Geometry check sheet. Reference: the model listing, model coordinates, mm. A direction names the side the tool comes from. Give positions to 0.01 mm unless a question says otherwise; leave off trailing zeros. Order: outer loops, then holes, each group sorted by start corner. A loop starts at its lowest first (then second) coordinate and runs counter-clockwise, first axis right, second up. Notation, with made-up numbers: M 59.25,4 L 89.25,4 A19 ccw 89.25,37 Z; hole C 2,-26.5 d9. An arc over 180 degrees is marked long. Put each result on its own line as item: value. Start each with the question number.
Q1. Section check C-C on y = -4.5. Record the cut outline in (x, z), then the cut area to 3 significant figures.
Q2. Access from +Z, -Z, +X, -X, +Y, -Y to the whole of each face (thin tool, end or side, straight path). Record for faces 4 (the flat face through (0, -6.172, 1)), 5 (the flat face through (0, -2.872, -0.3)), 6 (the flat face through (0, -2.872, 2.3)), 7 (the cylindrical face through (2.94, 1.9, 0.99)).
Q3. Section check A-A on y = 0. Record the cut outline in (x, z), then the cut area to 3 significant figures.
Q4. Mould release check, pull along Y, two halves, no side actions. Record for faces 1 (the conical face through (-0.031, -2.986, -0.964)), 2 (the cylindrical face through (0, -8, 0)), 3 (the cylindrical face through (-0.29, -2.23, 0.99)): +Y half, -Y half, draft (parallel to the pull), parting line (faces both ways), or undercut.
Q5. Section check D-D on z = 1. Record the cut outline in (x, y).
Q6. Section check B-B on z = 1.65. Record the cut outline in (x, y), then the cut area to 3 significant figures.
Q7. Go/stop test with flat-tipped pins: pin 1 (0.7 mm diameter, centred on x = 0, z = -0.5, fed in from +Y); pin 2 (1.6 mm diameter, centred on x = -0.5, z = 1, fed in from -Y); pin 3 (2 mm diameter, centred on y = -5.5, z = -1, fed in from -X); pin 4 (2 mm diameter, centred on y = -1.5, z = 1, fed in from +X). Record where each tip stops, or that it passes through.
Q8. Material ranges on L1, parallel to Z at x = 0, y = -6.9; L2, parallel to Y at x = 0, z = 1.4; L3, parallel to X at y = -0.75, z = 0.1, recorded low to high.
Autodesk Inventor part; units mm, degrees
ref_plane "YZ Plane" through (0, 0, 0) normal (1, 0, 0) x (0, 1, 0)
ref_plane "XZ Plane" through (0, 0, 0) normal (0, 1, 0) x (-1, 0, 0)
ref_plane "XY Plane" through (0, 0, 0) normal (0, 0, 1) x (1, 0, 0)
sketch "Sketch1" plane through (0, 0, 0) normal (0, 0, 1) x (1, 0, 0)
  circle A0 centre (0, 0) radius 2.25
  line L0 (0, 0) -> (0, -9.3774) construction
  line L1 (0, -9.3774) -> (2, -9.3774) construction
  line L2 (2, -9.3774) -> (2, -2.8723) construction
  circle A1 centre (0, 0) radius 3.5 construction
  line L3 (3.1465, -1.5328) -> (2, -4.6887)
  arc A2 (3.1465, -1.5328) -> (0, 3.5) centre (0, 0) ccw
  line L4 (-3.1465, -1.5328) -> (-2, -4.6887)
  arc A3 (0, 3.5) -> (-3.1465, -1.5328) centre (0, 0) ccw
  line L5 (2, -4.6887) -> (2, -2.8723)
  line L6 (-2, -4.6887) -> (-2, -2.8723)
  line L7 (-2, -2.8723) -> (2, -2.8723)
  dimension "d1" = 4.5
  dimension "d2" = 2
  dimension "d3" = 7
extrude "Extrusion1" add sketch "Sketch1" along normal blind 2
sketch "Sketch2" plane through (-2, -2.8723, 0) normal (0, -1, 0) x (1, 0, 0)
  line L0 (4, 2) -> (0, 2)
  line L1 (0, 0) -> (0, 2)
  line L2 (0, 0) -> (4, 0)
  line L3 (4, 0) -> (4, 2)
  line L4 (0, 2) -> (4, 0) construction
  line L5 (4, 2) -> (0, 0) construction
  circle A0 centre (2, 1) radius 2.25
  point P0 (2, 0)
  dimension "d6" = 4.5
extrude "Extrusion2" add sketch "Sketch2" along normal blind 6.3 contours L3 L2 L1 L0 | A0
sketch "Sketch3" plane through (0, -9.1723, 1) normal (0, -1, 0) x (1, 0, 0)
  circle A0 centre (0, 0) radius 2.25
  circle A1 centre (0, 0) radius 1
  point P0 (0, -1)
  dimension "d9" = 2
extrude "Extrusion3" cut sketch "Sketch3" against normal blind 3 contours A1
chamfer "Chamfer1" distance 0.4 angle 45 1 edges at (0, -2.8723, -1.25)
chamfer "Chamfer2" distance 0.4 angle 45 1 edges at (0, -2.8723, 3.25)
properties part number "union2"
Results found:
1. outline: M -2.07,0 L -2.02,0 A2.25 ccw 2.02,0 L 2.07,0 L 2.07,0.11 A2.25 ccw 2.07,1.89 L 2.07,2 L 2.02,2 A2.25 ccw -2.02,2 L -2.07,2 L -2.07,1.89 A2.25 ccw -2.07,0.11 Z
1. area: 15.9 mm^2
2. face 4: -Y
2. face 5: -Z, +X, -X, +Y
2. face 6: +Z, +X, -X, +Y
2. face 7: +Z, -Z, +X
3. outline: M -3.5,0 L -2.25,0 L -2.25,2 L -3.5,2 Z; M 2.25,0 L 3.5,0 L 3.5,2 L 2.25,2 Z
3. area: 5.00 mm^2
4. face 1: +Y half
4. face 2: draft
4. face 3: undercut
5. outline: M -3.15,-1.53 L -2.25,-4 L -2.25,-9.17 L -1,-9.17 L -1,-6.17 L 1,-6.17 L 1,-9.17 L 2.25,-9.17 L 2.25,-4 L 3.15,-1.53 A3.5 ccw 0,3.5 A3.5 ccw Z; hole C 0,0 d4.5
6. outline: M -3.15,-1.53 L -2.15,-4.26 L -2.15,-9.17 L -0.76,-9.17 L -0.76,-6.17 L 0.76,-6.17 L 0.76,-9.17 L 2.15,-9.17 L 2.15,-4.26 L 3.15,-1.53 A3.5 ccw 0,3.5 A3.5 ccw Z; hole C 0,0 d4.5
6. area: 44.8 mm^2
7. pin 1: stops at y = -2.87
7. pin 2: stops at y = -9.17
7. pin 3: stops at x = -2.02
7. pin 4: stops at x = 3.46
8. L1: z = -1.25 to 0, 2 to 3.25
8. L2: y = -6.17 to -2.25, 2.25 to 3.5
8. L3: x = -3.42 to -2.12, 2.12 to 3.42
